Source: CAD feature listing. Evaluate the final solid. Frame: model axes, mm. Face numbers are marked on the shaded views. Give positions to 0.01 mm unless a question says otherwise; leave off trailing zeros. Write each loop counter-clockwise with the first axis right and the second up, starting at its lowest first coordinate (ties: lowest second). Pieces come first, ordered by that corner, then holes. Notation, with made-up numbers: (83, 60.5) -> (100, 60.5) arc R17 ccw to (100, 71.5) -> close; hole circle Ø6 at (22.25, -24.5). An arc over 180 degrees is marked (long way). Use a Markdown table: item, result. Add a question column.
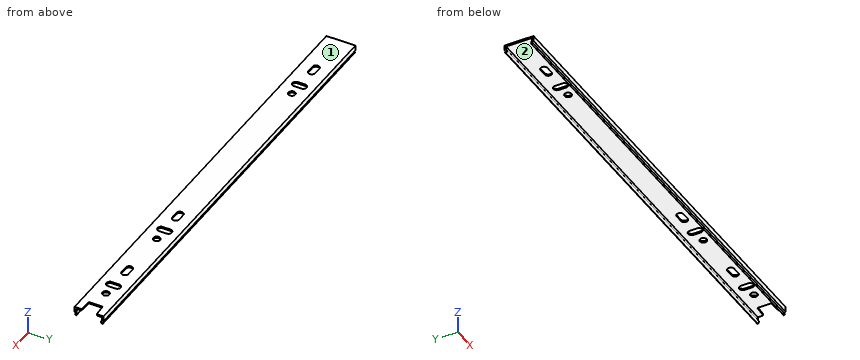
```python
from build123d import *

# Parameters (mm, degrees)
EXTRUDE_THIN1_DEPTH   = 298
ESBO_O1_R             = 2.25
CORTE_EXTRUS_O1_DEPTH = 299.207817733
FILETE1_R             = 0.5


with BuildPart() as part:
    # Sketch1 → Extrude-Thin1 (new body)
    with BuildSketch(Plane(origin=(0, 0, 0), x_dir=(0, 0, -1), z_dir=(1, 0, 0))):
        with BuildLine():
            ThreePointArc((-7.953264718, 8.5), (-9.353805922, 7.927754998), (-10.754347127, 8.5))
            Line((-10.754347127, 8.5), (-12.754347127, 8.5))
            Line((-12.754347127, 8.5), (-12.754347127, -8.5))
            Line((-12.754347127, -8.5), (-10.754347127, -8.5))
            ThreePointArc((-10.754347127, -8.5), (-9.353805922, -7.927754998), (-7.953264718, -8.5))
            Line((-7.953264718, -8.5), (-8.65353532, -9.213877499))
            ThreePointArc((-8.65353532, -9.213877499), (-9.529396971, -8.943291803), (-10.25770064, -9.5))
            Line((-10.25770064, -9.5), (-13.754347127, -9.5))
            Line((-13.754347127, -9.5), (-13.754347127, 9.5))
            Line((-13.754347127, 9.5), (-10.25770064, 9.5))
            ThreePointArc((-10.25770064, 9.5), (-9.529396971, 8.943291803), (-8.65353532, 9.213877499))
            Line((-8.65353532, 9.213877499), (-7.953264718, 8.5))
        make_face()
    extrude(amount=-EXTRUDE_THIN1_DEPTH)

    # Esboço1 → Corte-extrusão1 (cut, through all)
    with BuildSketch(Plane.XY.offset(13.754347127)):
        with Locations((-240, 0)):
            Circle(ESBO_O1_R)
        with Locations((-20, 0)):
            Circle(ESBO_O1_R)
        with Locations((-80, 0)):
            Circle(ESBO_O1_R)
        with BuildLine():
            Line((-268.425, 2.25), (-263.575, 2.25))
            ThreePointArc((-263.575, 2.25), (-261.325, 0), (-263.575, -2.25))
            Line((-263.575, -2.25), (-268.425, -2.25))
            ThreePointArc((-268.425, -2.25), (-270.675, 0), (-268.425, 2.25))
        make_face()
        with BuildLine():
            Line((-246.75, 2.425), (-246.75, -2.425))
            ThreePointArc((-246.75, -2.425), (-249, -4.675), (-251.25, -2.425))
            Line((-251.25, -2.425), (-251.25, 2.425))
            ThreePointArc((-251.25, 2.425), (-249, 4.675), (-246.75, 2.425))
        make_face()
        Polygon((-8, 4.5), (-8, -4.5), (0, -5), (0, 5), align=None)
        with BuildLine():
            Line((-47.425, 2.25), (-42.575, 2.25))
            ThreePointArc((-42.575, 2.25), (-40.325, 0), (-42.575, -2.25))
            Line((-42.575, -2.25), (-47.425, -2.25))
            ThreePointArc((-47.425, -2.25), (-49.675, 0), (-47.425, 2.25))
        make_face()
        with BuildLine():
            Line((-26.75, 2.425), (-26.75, -2.425))
            ThreePointArc((-26.75, -2.425), (-29, -4.675), (-31.25, -2.425))
            Line((-31.25, -2.425), (-31.25, 2.425))
            ThreePointArc((-31.25, 2.425), (-29, 4.675), (-26.75, 2.425))
        make_face()
        with BuildLine():
            Line((-107.425, 2.25), (-102.575, 2.25))
            ThreePointArc((-102.575, 2.25), (-100.325, 0), (-102.575, -2.25))
            Line((-102.575, -2.25), (-107.425, -2.25))
            ThreePointArc((-107.425, -2.25), (-109.675, 0), (-107.425, 2.25))
        make_face()
        with BuildLine():
            Line((-87.25, 2.425), (-87.25, -2.425))
            ThreePointArc((-87.25, -2.425), (-89.5, -4.675), (-91.75, -2.425))
            Line((-91.75, -2.425), (-91.75, 2.425))
            ThreePointArc((-91.75, 2.425), (-89.5, 4.675), (-87.25, 2.425))
        make_face()
    extrude(amount=-CORTE_EXTRUS_O1_DEPTH, mode=Mode.SUBTRACT)

    # Filete1
    filete1_edges = [part.edges().sort_by_distance(p)[0] for p in [
        (-8, -4.5, 13.254347127),
        (-8, 4.5, 13.254347127),
        (0, 5, 13.254347127),
        (0, -5, 13.254347127),
    ]]
    fillet(filete1_edges, radius=FILETE1_R)


solid = part.part
```
(1) Cut plane A-A on x = -146. Return the cut outline in (y, z).
(2) Material intervals for L1, parallel to Y at x = -80, z = 13.25; L2, parallel to Y at x = -95.5, z = 12.4; L3, parallel to Z at x = -258.5, y = -1, sorted ascending.
(3) Mould query, pull axis Y, two halves, no side actions, for the marked faces 1 and 2. Classes: +Y half, -Y half, draft (parallel to the pull), parting line (faces both ways), or undercut.
(4) First-contact query: pin 1 Ø0.5 at (y, z) = (-1, 13) entering from +X; pin 2 Ø1 at (x, y) = (-226.5, -3.5) entering from -Z. Flat tips, straight axial feed; report the tip coordinate or a pass-through.
Output:
| question | item | result |
|---|---|---|
| 1 | outline | (-9.5, 10.26) arc R1 cw to (-9.21, 8.65) -> (-8.5, 7.95) arc R2 ccw to (-8.5, 10.75) -> (-8.5, 12.75) -> (8.5, 12.75) -> (8.5, 10.75) arc R2 ccw to (8.5, 7.95) -> (9.21, 8.65) arc R1 cw to (9.5, 10.26) -> (9.5, 13.75) -> (-9.5, 13.75) -> close |
| 2 | L1 | -9.5 to -2.25, 2.25 to 9.5 |
| 2 | L2 | -9.5 to -8.5, 8.5 to 9.5 |
| 2 | L3 | 12.75 to 13.75 |
| 3 | face 1 | draft |
| 3 | face 2 | undercut |
| 4 | pin 1 | x = -8 |
| 4 | pin 2 | z = 12.75 |
